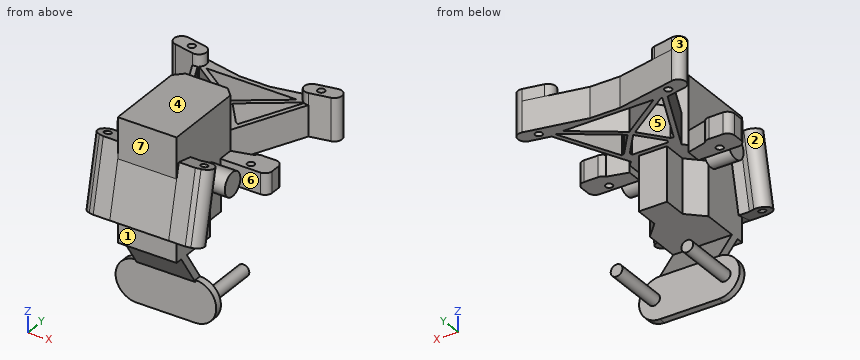
from build123d import *

# Parameters (mm, degrees)
SKETCH1_R                    = 5
DRIVELINE_AXIS_DEPTH         = 23
DUMMY_BOSS_DEPTH             = 26
SKETCH8_R                    = 1.5
UPRIGHTS_DEPTH               = 10
UPRIGHTS_DEPTH_BACK          = 3
SKETCH9_R                    = 1.5
SHOCK_MOUNT_DEPTH            = 5
SHOCK_MOUNT_DEPTH_BACK       = 13
SKETCH10_R                   = 1.5
TURNBUCKLE_MOUNTS_DEPTH      = 3
TURNBUCKLE_MOUNTS_DEPTH_BACK = 6
TURNBUCKLE_ROOM_DEPTH        = 1
TURNBUCKLE_ROOM_DEPTH_BACK   = 23
BOSS_EXTRUDE2_DEPTH          = 12.5
BOSS_EXTRUDE3_DEPTH          = 3
SKETCH43_R                   = 2.5
BOSS_EXTRUDE4_DEPTH          = 24
BOSS_EXTRUDE5_DEPTH          = 15
BOSS_EXTRUDE6_DEPTH          = 12.5
SKETCH49_R                   = 1.5
CUT_EXTRUDE1_DEPTH           = 15


with BuildPart() as part:
    # Sketch1 → Driveline Axis (new body, symmetric)
    with BuildSketch(Plane(origin=(0, 0, 0), x_dir=(0, 0, -1), z_dir=(1, 0, 0))):
        Circle(SKETCH1_R)
    extrude(amount=DRIVELINE_AXIS_DEPTH, both=True)

    # Sketch2 → Dummy Boss (add, symmetric)
    with BuildSketch(Plane.XY):
        Polygon((-12.5, -20), (-12.5, 14.464466094), (-8.964466094, 18), (8.964466094, 18), (12.5, 14.464466094), (12.5, -20), align=None)
    extrude(amount=DUMMY_BOSS_DEPTH, both=True)

    # Sketch8 → Uprights (add, two sides)
    with BuildSketch(Plane.XY) as uprights_sk:
        with BuildLine():
            Line((-10.732233047, 16.232233047), (-24.661465898, 46.103569293))
            Line((-24.661465898, 46.103569293), (-33.048979486, 47.815663334))
            ThreePointArc((-33.048979486, 47.815663334), (-35.583316151, 51.65), (-31.748979486, 54.184336666))
            Line((-31.748979486, 54.184336666), (-6.351020514, 49))
            Line((-6.351020514, 49), (6.351020514, 49))
            Line((6.351020514, 49), (31.748979486, 54.184336666))
            ThreePointArc((31.748979486, 54.184336666), (35.583316151, 51.65), (33.048979486, 47.815663334))
            Line((33.048979486, 47.815663334), (24.661465898, 46.103569293))
            Line((24.661465898, 46.103569293), (10.732233047, 16.232233047))
            Line((10.732233047, 16.232233047), (8.964466094, 18))
            Line((8.964466094, 18), (-8.964466094, 18))
            Line((-8.964466094, 18), (-10.732233047, 16.232233047))
        make_face()
        with Locations((-27.5, 50)):
            Circle(SKETCH8_R, mode=Mode.SUBTRACT)
        with Locations((27.5, 50)):
            Circle(SKETCH8_R, mode=Mode.SUBTRACT)
        with BuildLine():
            Line((9.866245938, 21.994232403), (1.612099151, 32.1872548))
            Line((1.612099151, 32.1872548), (22.924030195, 47.110029571))
            Line((22.924030195, 47.110029571), (10.997739753, 21.534017182))
            ThreePointArc((10.997739753, 21.534017182), (10.467987263, 21.852621345), (9.866245938, 21.994232403))
        make_face(mode=Mode.SUBTRACT)
        with BuildLine():
            Line((7.714466094, 20), (-7.714466094, 20))
            ThreePointArc((-7.714466094, 20), (-7.795487149, 20.563488959), (-8.031985901, 21.081323449))
            Line((-8.031985901, 21.081323449), (0, 31))
            Line((0, 31), (8.031985901, 21.081323449))
            ThreePointArc((8.031985901, 21.081323449), (7.795487149, 20.563488959), (7.714466094, 20))
        make_face(mode=Mode.SUBTRACT)
        with BuildLine():
            Line((-10.997739753, 21.534017182), (-22.924030195, 47.110029571))
            Line((-22.924030195, 47.110029571), (-1.612099151, 32.1872548))
            Line((-1.612099151, 32.1872548), (-9.866245938, 21.994232403))
            ThreePointArc((-9.866245938, 21.994232403), (-10.467987263, 21.852621345), (-10.997739753, 21.534017182))
        make_face(mode=Mode.SUBTRACT)
        Polygon((-19.279998091, 47), (0, 33.5), (19.279998091, 47), align=None, mode=Mode.SUBTRACT)
    extrude(amount=UPRIGHTS_DEPTH)
    extrude(uprights_sk.sketch, amount=-UPRIGHTS_DEPTH_BACK)

    # Sketch9 → Shock Mount (add, two sides)
    with BuildSketch(Plane.XY.offset(10)) as shock_mount_sk:
        with BuildLine():
            Line((-24.661465898, 46.103569293), (-33.048979486, 47.815663334))
            ThreePointArc((-33.048979486, 47.815663334), (-35.583316151, 51.65), (-31.748979486, 54.184336666))
            Line((-31.748979486, 54.184336666), (-23.361465898, 52.472242624))
            ThreePointArc((-23.361465898, 52.472242624), (-20.827129232, 48.637905958), (-24.661465898, 46.103569293))
        make_face()
        with Locations((-27.5, 50)):
            Circle(SKETCH9_R, mode=Mode.SUBTRACT)
        with BuildLine():
            Line((23.361465898, 52.472242624), (31.748979486, 54.184336666))
            ThreePointArc((31.748979486, 54.184336666), (35.583316151, 51.65), (33.048979486, 47.815663334))
            Line((33.048979486, 47.815663334), (24.661465898, 46.103569293))
            ThreePointArc((24.661465898, 46.103569293), (20.827129232, 48.637905958), (23.361465898, 52.472242624))
        make_face()
        with Locations((27.5, 50)):
            Circle(SKETCH9_R, mode=Mode.SUBTRACT)
    extrude(amount=SHOCK_MOUNT_DEPTH)
    extrude(shock_mount_sk.sketch, amount=-SHOCK_MOUNT_DEPTH_BACK)

    # Sketch10 → Turnbuckle Mounts (add, two sides)
    with BuildSketch(Plane.XY) as turnbuckle_mounts_sk:
        with BuildLine():
            Line((29.5, 8), (12.5, 8))
            Line((12.5, 8), (12.5, 14.464466094))
            Line((12.5, 14.464466094), (21.055616084, 16.739249053))
            ThreePointArc((21.055616084, 16.739249053), (22.124817677, 17.666247097), (23.5, 18))
            Line((23.5, 18), (29.5, 18))
            ThreePointArc((29.5, 18), (31.621320344, 17.121320344), (32.5, 15))
            Line((32.5, 15), (32.5, 11))
            ThreePointArc((32.5, 11), (31.621320344, 8.878679656), (29.5, 8))
        make_face()
        with Locations((23.5, 11)):
            Circle(SKETCH10_R, mode=Mode.SUBTRACT)
        with BuildLine():
            Line((-12.5, 14.464466094), (-21.055616084, 16.739249053))
            ThreePointArc((-21.055616084, 16.739249053), (-22.124817677, 17.666247097), (-23.5, 18))
            Line((-23.5, 18), (-29.5, 18))
            ThreePointArc((-29.5, 18), (-31.621320344, 17.121320344), (-32.5, 15))
            Line((-32.5, 15), (-32.5, 11))
            ThreePointArc((-32.5, 11), (-31.621320344, 8.878679656), (-29.5, 8))
            Line((-29.5, 8), (-12.5, 8))
            Line((-12.5, 8), (-12.5, 14.464466094))
        make_face()
        with Locations((-23.5, 11)):
            Circle(SKETCH10_R, mode=Mode.SUBTRACT)
    extrude(amount=TURNBUCKLE_MOUNTS_DEPTH)
    extrude(turnbuckle_mounts_sk.sketch, amount=-TURNBUCKLE_MOUNTS_DEPTH_BACK)

    # Sketch11 → Turnbuckle Room (cut, two sides)
    with BuildSketch(Plane(origin=(0, 0, -26), x_dir=(-1, 0, 0), z_dir=(0, 0, -1))) as turnbuckle_room_sk:
        Polygon((8.964466094, 18), (5.75, 18), (5.75, 8), (12.5, 1.544903812), (12.5, 14.464466094), align=None)
        Polygon((-12.5, 14.464466094), (-12.5, 1.464466094), (-6.25, 8), (-6.25, 18), (-8.964466094, 18), align=None)
    extrude(amount=TURNBUCKLE_ROOM_DEPTH, mode=Mode.SUBTRACT)
    extrude(turnbuckle_room_sk.sketch, amount=-TURNBUCKLE_ROOM_DEPTH_BACK, mode=Mode.SUBTRACT)

    # Sketch40 → Boss-Extrude2 (add, symmetric)
    with BuildSketch(Plane(origin=(0, 0, 0), x_dir=(0, 0, -1), z_dir=(1, 0, 0))):
        Polygon((26, -13.433574933), (39.118894341, -5), (56.881105659, -5), (56.881105659, -8), (40, -8), (26, -17), align=None)
    extrude(amount=BOSS_EXTRUDE2_DEPTH, both=True)

    # Sketch41 → Boss-Extrude3 (add)
    with BuildSketch(Plane(origin=(0, -5, 0), x_dir=(1, 0, 0), z_dir=(0, 1, 0))):
        with BuildLine():
            Line((12.5, 56.881105659), (12.5, 39.118894341))
            ThreePointArc((12.5, 39.118894341), (21.381105659, 48), (12.5, 56.881105659))
        make_face()
    boss_extrude3 = extrude(amount=-BOSS_EXTRUDE3_DEPTH)

    # Mirror4: Boss-Extrude3 across plane
    add(boss_extrude3.mirror(Plane(origin=(0, 0, 0), x_dir=(0, 0, 1), z_dir=(1, 0, 0))))

    # Sketch43 → Boss-Extrude4 (add)
    with BuildSketch(Plane(origin=(0, -5, 0), x_dir=(1, 0, 0), z_dir=(0, 1, 0))):
        with Locations((-15, 48)):
            Circle(SKETCH43_R)
        with Locations((15, 48)):
            Circle(SKETCH43_R)
    extrude(amount=BOSS_EXTRUDE4_DEPTH)

    # Sketch47 → Boss-Extrude5 (add, symmetric)
    with BuildSketch(Plane(origin=(0, -0.93692213, -4.226182617), x_dir=(0, 0.976296007, -0.216439614), z_dir=(0, -0.216439614, -0.976296007))):
        with BuildLine():
            Line((-13.806627078, 12.5), (-13.806627078, 17.084049145))
            Line((-13.806627078, 17.084049145), (-13.149862777, 19.41536026))
            ThreePointArc((-13.149862777, 19.41536026), (-15.91536026, 24.350137223), (-20.850137223, 21.58463974))
            Line((-20.850137223, 21.58463974), (-21.423285097, 19.550141201))
            Line((-21.423285097, 19.550141201), (-21.423285097, 12.5))
            Line((-21.423285097, 12.5), (-13.806627078, 12.5))
        make_face()
    boss_extrude5 = extrude(amount=BOSS_EXTRUDE5_DEPTH, both=True)

    # Sketch48 → Boss-Extrude6 (add)
    with BuildSketch(Plane.ZY.offset(-12.5)):
        Polygon((-14.233775168, -25.098984039), (8.766255495, -20), (-15.364192715, -20), align=None)
    boss_extrude6 = extrude(amount=BOSS_EXTRUDE6_DEPTH)

    # Sketch49 → Cut-Extrude1 (cut, symmetric)
    with BuildSketch(Plane(origin=(0, -0.93692213, -4.226182617), x_dir=(0, 0.976296007, -0.216439614), z_dir=(0, -0.216439614, -0.976296007))):
        with Locations((-17, 20.5)):
            Circle(SKETCH49_R)
    cut_extrude1 = extrude(amount=CUT_EXTRUDE1_DEPTH, both=True, mode=Mode.SUBTRACT)

    # Mirror5: Boss-Extrude5, Boss-Extrude6, Cut-Extrude1 across plane
    add(boss_extrude5.mirror(Plane(origin=(0, 0, 0), x_dir=(0, 0, 1), z_dir=(1, 0, 0))))
    add(boss_extrude6.mirror(Plane(origin=(0, 0, 0), x_dir=(0, 0, 1), z_dir=(1, 0, 0))))
    add(cut_extrude1.mirror(Plane(origin=(0, 0, 0), x_dir=(0, 0, 1), z_dir=(1, 0, 0))), mode=Mode.SUBTRACT)


solid = part.part
Work out the finished part from the listing and answer in its coordinate system (mm). Face numbers are marked on the shaded views. A direction names the side the tool comes from. Round coordinates to 2 decimals unless told otherwise and drop trailing zeros. Order: outer loops, then holes, each group sorted by start corner. A loop starts at its lowest first (then second) coordinate and runs counter-clockwise, first axis right, second up. Notation, with made-up numbers: M 47,-4 L 75,-4 A21 cw 75,22 Z; hole C 37,-19.75 d2. An arc over 180 degrees is marked long. Put each result on its own line as item: value. Start each with the question number.
Q1. Section C-C, the plane z = -19 is taken. Write down the section's boundary in (x, y), and give its area (3 significant figures).
Q2. Flat-ended cylindrical pins translate along their axes: pin 1 (6.5 mm diameter, centred on x = 25.5, z = -1.5, fed in from +Y); pin 2 (2.5 mm diameter, centred on x = 27.5, y = 50, fed in from +Z); pin 3 (5 mm diameter, centred on x = -23.5, y = 11, fed in from -Z); pin 4 (2.5 mm diameter, centred on x = -15, z = -48.5, fed in from +Y). Find the tip coordinate at first contact, or state that the pin passes through.
Q3. Straight lines are drawn through the part: L1, parallel to Y at x = -23.5, z = -1.25; L2, parallel to Y at x = 27.5, z = 1.25; L3, parallel to Y at x = -23.5, z = -3.75. For each, find the intervals that lie inside material, in ascending order. Write a range as [from, to].
Q4. Section B-B, the plane x = 14 is taken. Give the number of separate pieces and of enclosed holes in the cut face, and give its area (3 significant figures).
Q5. For a pull along Y with two mould halves and no side action, classify the marked faces 1, 2, 3 and 4 as pulls with the +Y half, pulls with the -Y half, needs draft (parallel to the pull), parting line crosses it, or undercut.
Q6. Section A-A, the plane y = -3 is taken. Write down the section's boundary in (x, z).
Q7. A tool of negligible diameter and unlimited length cuts with its end or side. For the marked faces 5, 6 and 7, from which of +Z, -Z, +X, -X, +Y, -Y can it reach the whole face along a straight path? Write none if from no direction.
Findings below:
1. outline: M -12.5,-20 L 12.5,-20 L 12.5,1.46 L 6.25,8 L 6.25,18 L -5.75,18 L -5.75,8 L -12.5,1.54 Z
1. area: 778 mm^2
2. pin 1: stops at y = 53.57
2. pin 2: passes through
2. pin 3: stops at z = -6
2. pin 4: stops at y = 19
3. L1: y = [-20.4, -14.98], [8, 9.5], [12.5, 18], [43.61, 52.5]
3. L2: y = [8, 18], [46.68, 48.5], [51.5, 53.32]
3. L3: y = [-20.95, -15.53], [8, 9.5], [12.5, 18]
4. separate pieces: 7
4. enclosed holes: 0
4. area: 671 mm^2
5. face 1: pulls with the -Y half
5. face 2: undercut
5. face 3: parting line crosses it
5. face 4: needs draft
6. outline: M -23,-4 L -12.5,-4 L -12.5,-26 L 12.5,-26 L 12.5,-4 L 23,-4 L 23,4 L 12.5,4 L 12.5,26 L -12.5,26 L -12.5,4 L -23,4 Z; C -15,-48 d5; C 15,-48 d5
7. face 5: +Z, -Z
7. face 6: +Z, +X
7. face 7: +Z, +X, -X, -Y
